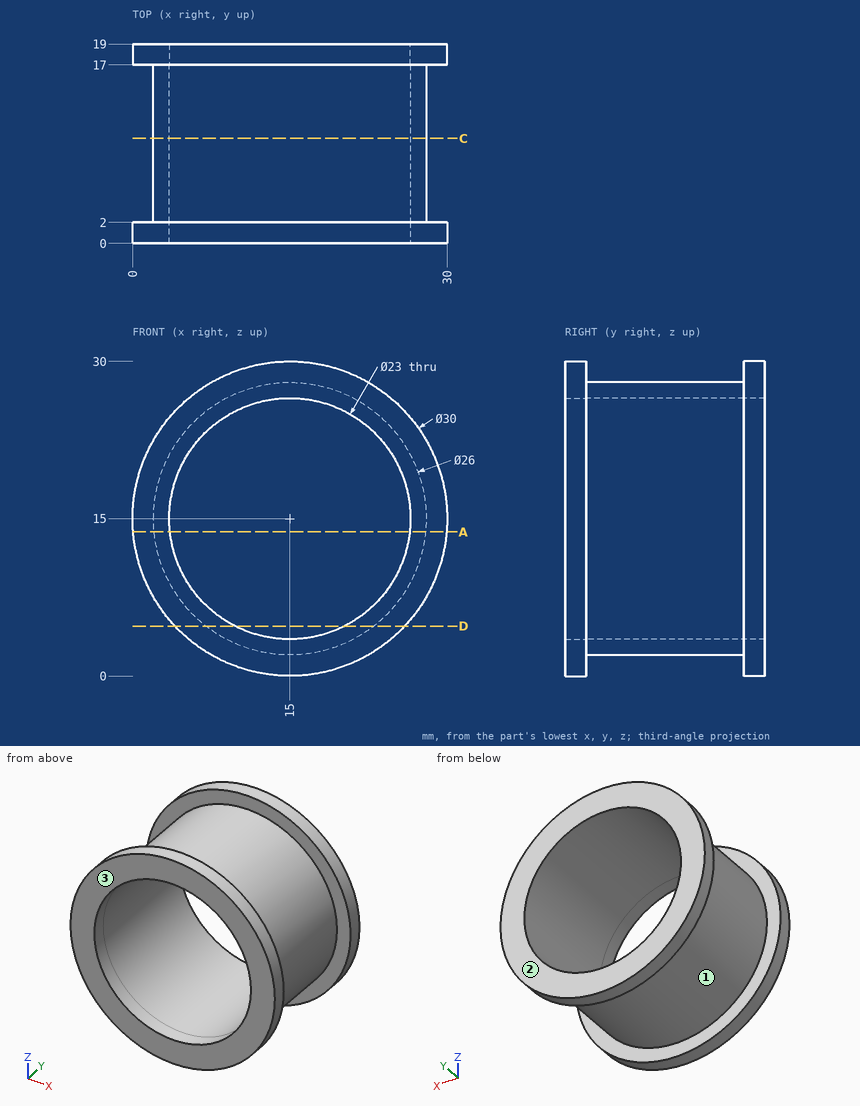
Job drawing, mm, ordinate dimensions from the low corner. One solid piece. Give positions to 0.01 mm unless a question says otherwise; leave off trailing zeros. Order: outer loops, then holes, each group sorted by start corner. A loop starts at its lowest first (then second) coordinate and runs counter-clockwise, first axis right, second up. Notation, with made-up numbers: M 33,-23.5 L 81,-23.5 A17 cw 81,-14.5 Z; hole C 17.25,82 d8. An arc over 180 degrees is marked long. Put each result on its own line as item: value. Start each with the question number.
(1) Band-saw the part on D-D on z = 4.75. Give the cut face in (x, y), then the cut area to 3 significant figures.
(2) Drill centre lines: L1, parallel to Y at x = 20.5, z = 2.75; L2, parallel to Z at x = 15, y = 15.25. Where is each one in solid material? Low to high. Write a range as [from, to].
(3) Pull direction Y, two halves, no side cores. Call the marked faces 1, 2 and 3: released by +Y, released by -Y, zero draft, split by the parting line, or undercut.
(4) Pin check, flat tips, straight feed: pin 1 Ø5 at (y, z) = (5.5, 17.5) entering from +X; pin 2 Ø8 at (x, y) = (7.5, 10.5) entering from -Z; pin 3 Ø8 at (x, y) = (10, 2.5) entering from +Z; pin 4 Ø1 at (x, z) = (19.5, 5) entering from +Y. Stop position of each tip, or through.
(5) Band-saw the part on A-A on z = 13.75. Give the cut face in (x, y).
(6) Band-saw the part on C-C on y = 10. Give the cut face in (x, z), then the cut area to 3 significant figures.
Results below:
1. outline: M 4.05,0 L 9.79,0 L 9.79,19 L 4.05,19 L 4.05,17 L 7,17 L 7,2 L 4.05,2 Z; M 20.21,0 L 25.95,0 L 25.95,2 L 23,2 L 23,17 L 25.95,17 L 25.95,19 L 20.21,19 Z
1. area: 129 mm2
2. L1: y = [0, 2], [17, 19]
2. L2: z = [2, 3.5], [26.5, 28]
3. face 1: undercut
3. face 2: released by +Y
3. face 3: released by -Y
4. pin 1: stops at x = 28
4. pin 2: stops at z = 2.48
4. pin 3: stops at z = 29.96
4. pin 4: passes through
5. outline: M 0.05,0 L 3.57,0 L 3.57,19 L 0.05,19 L 0.05,17 L 2.06,17 L 2.06,2 L 0.05,2 Z; M 26.43,0 L 29.95,0 L 29.95,2 L 27.94,2 L 27.94,17 L 29.95,17 L 29.95,19 L 26.43,19 Z
6. outline: C 15,15 d26; hole C 15,15 d23
6. area: 115 mm2
